```python
from build123d import *

# Parameters (mm, degrees)
F1_DEPTH = 10
F0_W     = 3.383045
F0_H     = 2
F2_DEPTH = 5


with BuildPart() as f1:
    # F0 (on Front) → F1 (new body, symmetric)
    with BuildSketch(Plane.XZ):
        Polygon((-69.820315, 2), (-69.820315, 0), (-44.373278, 0), (-44.373278, 2), (-49.617426, 2), (-55.793015, 2), (-58.917426, 2), (-65.093015, 2), align=None)
    extrude(amount=F1_DEPTH, both=True)

    # F0 (on Front) → F2 (join, symmetric)
    with BuildSketch(Plane.XZ):
        Polygon((-55.793015, 2), (-49.617426, 2), (-49.617426, 10), (-50.923162, 10), (-54.306207, 10), (-55.793015, 10), align=None)
        Polygon((-65.093015, 10), (-65.093015, 2), (-58.917426, 2), (-58.917426, 10), (-60.223162, 10), (-63.606207, 10), align=None)
        Polygon((-65.093017, 22), (-63.606208, 22), (-60.223163, 22), (-58.917428, 22), (-58.917428, 30), (-60.223164, 30), (-63.606209, 30), (-65.093017, 30), align=None)
        Polygon((-65.093018, 32), (-63.606209, 32), (-60.223164, 32), (-58.917429, 32), (-58.917429, 40), (-60.223165, 40), (-63.60621, 40), (-65.093018, 40), align=None)
        with Locations((-61.914687, 31)):
            Rectangle(F0_W, F0_H)
        with Locations((-52.614688, 51)):
            Rectangle(F0_W, F0_H)
        with Locations((-61.914685, 21)):
            Rectangle(F0_W, F0_H)
        with Locations((-52.614684, 11)):
            Rectangle(F0_W, F0_H)
        Polygon((-54.30621, 42), (-50.923165, 42), (-49.61743, 42), (-49.61743, 50), (-50.923166, 50), (-54.306211, 50), (-55.793019, 50), (-55.793019, 42), align=None)
        Polygon((-65.093019, 42), (-63.60621, 42), (-60.223165, 42), (-58.91743, 42), (-58.91743, 50), (-60.223166, 50), (-63.606211, 50), (-65.093019, 50), align=None)
        with Locations((-61.914684, 11)):
            Rectangle(F0_W, F0_H)
        with Locations((-52.614688, 41)):
            Rectangle(F0_W, F0_H)
        Polygon((-54.306209, 32), (-50.923164, 32), (-49.617429, 32), (-49.617429, 40), (-50.923165, 40), (-54.30621, 40), (-55.793018, 40), (-55.793018, 32), align=None)
        Polygon((-54.306207, 12), (-50.923162, 12), (-49.617427, 12), (-49.617427, 20), (-50.923163, 20), (-54.306208, 20), (-55.793016, 20), (-55.793016, 12), align=None)
        Polygon((-54.306208, 22), (-50.923163, 22), (-49.617428, 22), (-49.617428, 30), (-50.923164, 30), (-54.306209, 30), (-55.793017, 30), (-55.793017, 22), align=None)
        with Locations((-52.614686, 31)):
            Rectangle(F0_W, F0_H)
        Polygon((-65.093016, 12), (-63.606207, 12), (-60.223162, 12), (-58.917427, 12), (-58.917427, 20), (-60.223163, 20), (-63.606208, 20), (-65.093016, 20), align=None)
        Polygon((-54.306211, 52), (-50.923166, 52), (-49.617431, 52), (-49.617431, 60), (-50.923167, 60), (-54.306212, 60), (-55.79302, 60), (-55.79302, 52), align=None)
        with Locations((-61.914688, 51)):
            Rectangle(F0_W, F0_H)
        with Locations((-61.914687, 41)):
            Rectangle(F0_W, F0_H)
        with Locations((-52.614685, 21)):
            Rectangle(F0_W, F0_H)
        Polygon((-65.09302, 52), (-63.606211, 52), (-60.223166, 52), (-58.917431, 52), (-58.917431, 60), (-60.223167, 60), (-63.606212, 60), (-65.09302, 60), align=None)
    extrude(amount=F2_DEPTH, both=True)


solid = f1.part
```
Design review of the part built by this model. Coordinates are the model's own, in mm. A direction names the side the tool comes from. Give positions to 0.01 mm unless a question says otherwise; leave off trailing zeros. Loops run counter-clockwise (first coordinate to the right, second up) from the corner with the lowest first, then second, coordinate; pieces in that order, holes last. Notation, with made-up numbers: M 44,-34 L 73,-34 A25 ccw 73,-11 Z; hole C -21,44.5 d10. An arc over 180 degrees is marked long. Return JSON: item names as keys, results as strings. Group by question number.
Item 1: We need section C-C (y = -6.5). Give the boundary of the cut face in (x, z), and give its area (3 significant figures).
Item 2: Mouldability with a two-part tool opening along Z and no side actions: class faces 4 (the flat face through (-50.923, 0, 11)), 5 (the flat face through (-65.093, 0, 26)) as released by +Z, released by -Z, zero draft, split by the parting line, or undercut.
Item 3: Tool access review of faces 1 (the flat face through (-50, 0, 20)), 2 (the flat face through (-49.617, 0, 46)), 3 (the flat face through (-60.223, 0, 41)): name each direction out of +Z, -Z, +X, -X, +Y, -Y from which nothing blocks a thin tool from reaching the whole face with its end or side.
Item 4: We need section A-A (z = 5). Give the boundary of the cut face in (x, y), and give its area (3 significant figures).
Item 5: We need section B-B (x = -62.75). Give the boundary of the cut face in (y, z).
Item 6: We need section D-D (x = -46.25). Give the boundary of the cut face in (y, z), and give its area (3 significant figures).
Item 7: For probe 1 along Z at (x, y) = (-59.75, -1.5); probe 2 along X at (y, z) = (-4, 5.5); probe 3 along Z at (x, y) = (-57.5, -0.5), list the stretches that pass through material, from the lowest coordinate up.
Item 8: Insertion check: pin 1 Ø2 at (y, z) = (-3, 50.5) entering from -X; pin 2 Ø9 at (y, z) = (-2.5, 46) entering from +X; pin 3 Ø5 at (x, y) = (-64.5, -8) entering from -Z; pin 4 Ø6 at (x, z) = (-51.5, 11) entering from +Y. Each pin has a flat end and moves straight along its axis. Give the tip position at first contact, or say it passes through.
Output:
{
 "1": {"outline": "M -69.82,0 L -44.37,0 L -44.37,2 L -69.82,2 Z", "area": "50.9 mm^2"},
 "2": {"face 4": "undercut", "face 5": "zero draft"},
 "3": {"face 1": "+X, +Y, -Y", "face 2": "+Z, +X, +Y, -Y", "face 3": "+Y, -Y"},
 "4": {"outline": "M -65.09,-5 L -58.92,-5 L -58.92,5 L -65.09,5 Z; M -55.79,-5 L -49.62,-5 L -49.62,5 L -55.79,5 Z", "area": "124 mm^2"},
 "5": {"outline": "M -10,0 L 10,0 L 10,2 L 5,2 L 5,60 L -5,60 L -5,2 L -10,2 Z"},
 "6": {"outline": "M -10,0 L 10,0 L 10,2 L -10,2 Z", "area": "40.0 mm^2"},
 "7": {"probe 1": "z = 0 to 10, 12 to 20, 22 to 30, 32 to 40, 42 to 50, 52 to 60", "probe 2": "x = -65.09 to -58.92, -55.79 to -49.62", "probe 3": "z = 0 to 2"},
 "8": {"pin 1": "stops at x = -65.09", "pin 2": "stops at x = -49.62", "pin 3": "stops at z = 0", "pin 4": "stops at y = 5"}
}
